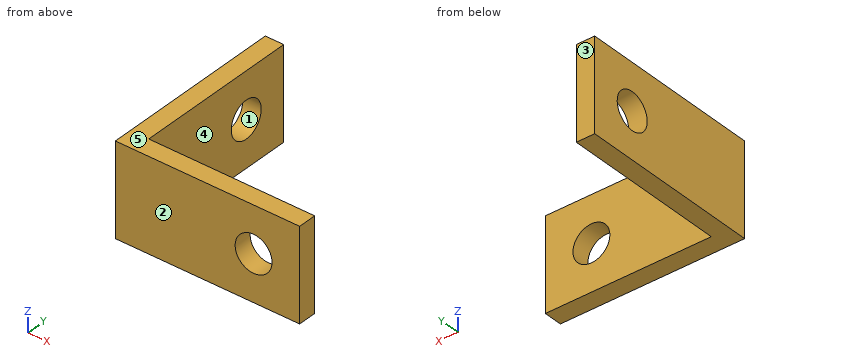
from build123d import *

# Parameters (mm, degrees)
SKETCH1_W           = 2
SKETCH1_H           = 18
SKETCH1_H_2         = 2
SKETCH1_W_2         = 18
BOSS_EXTRUDE2_DEPTH = 10
SKETCH3_R           = 2
CUT_EXTRUDE1_DEPTH  = 3
SKETCH4_R           = 2
CUT_EXTRUDE2_DEPTH  = 3


with BuildPart() as part:
    # Sketch1 → Boss-Extrude2 (new body)
    with BuildSketch(Plane.XY):
        with Locations((-8.840572317, 11)):
            Rectangle(SKETCH1_W, SKETCH1_H)
        with Locations((-8.840572317, 1)):
            Rectangle(SKETCH1_W, SKETCH1_H_2)
        with Locations((1.159427683, 1)):
            Rectangle(SKETCH1_W_2, SKETCH1_H_2)
    extrude(amount=BOSS_EXTRUDE2_DEPTH)

    # Sketch3 → Cut-Extrude1 (cut, through all)
    with BuildSketch(Plane(origin=(0, 2, 0), x_dir=(1, 0, 0), z_dir=(0, 1, 0))):
        with Locations((5.159427683, -5)):
            Circle(SKETCH3_R)
    extrude(amount=-CUT_EXTRUDE1_DEPTH, mode=Mode.SUBTRACT)

    # Sketch4 → Cut-Extrude2 (cut, through all)
    with BuildSketch(Plane(origin=(-7.840572317, 0, 0), x_dir=(0, 0, -1), z_dir=(1, 0, 0))):
        with Locations((-5, 15)):
            Circle(SKETCH4_R)
    extrude(amount=-CUT_EXTRUDE2_DEPTH, mode=Mode.SUBTRACT)


solid = part.part
Could you check a few things on this model? Use its own coordinates, in mm. Face numbers are marked on the shaded views. A direction names the side the tool comes from. Coordinates: 2 decimals unless noted, no trailing zeros. Loops run counter-clockwise (first coordinate to the right, second up) from the corner with the lowest first, then second, coordinate; pieces in that order, holes last.
1. Imagine slicing it at D-D (x = -6.5). Please give me the cut outline in (y, z), and give its area (3 significant figures).
2. For P1, Ø3, axis at y = 11, z = 6.5, coming from the +X side; P2, Ø12, axis at x = 4.5, y = 6, coming from the +Z side, each with a flat end and sliding along its axis, tell me the tip position at first contact or that it passes through.
3. Imagine slicing it at A-A (z = 5). Please give me the cut outline in (x, y), and give its area (3 significant figures).
4. Imagine slicing it at C-C (z = 8.25). Please give me the cut outline in (x, y), and give its area (3 significant figures).
5. We'd pull the mould along Y, two halves only. Please class the marked faces 1, 2 and 3: released by +Y, released by -Y, zero draft, split by the parting line, or undercut.
6. I need wall thicknesses on L1, parallel to X at y = 1.25, z = 5; L2, parallel to Y at x = -8.5, z = 5; L3, parallel to X at y = 19.25, z = 0.75. Which ranges of each line are inside material? Lowest first, please.
7. For the marked faces 4 and 5, which set-ups out of +Z, -Z, +X, -X, +Y, -Y let a thin tool reach every point of the face, with its end or its side?
8. Imagine slicing it at B-B (y = 15). Please give me the cut outline in (x, z).
Computed values:
1. outline: (0, 0) - (2, 0) - (2, 10) - (0, 10) - close
1. area: 20.0 mm2
2. P1: stops at x = -7.84
2. P2: stops at z = 10
3. outline: (-9.84, 0) - (3.16, 0) - (3.16, 2) - (-7.84, 2) - (-7.84, 13) - (-9.84, 13) - close; (-9.84, 17) - (-7.84, 17) - (-7.84, 20) - (-9.84, 20) - close; (7.16, 0) - (10.16, 0) - (10.16, 2) - (7.16, 2) - close
3. area: 60.0 mm2
4. outline: (-9.84, 0) - (10.16, 0) - (10.16, 2) - (-7.84, 2) - (-7.84, 20) - (-9.84, 20) - close
4. area: 76.0 mm2
5. face 1: undercut
5. face 2: released by -Y
5. face 3: released by +Y
6. L1: x = -9.84 to 3.16, 7.16 to 10.16
6. L2: y = 0 to 13, 17 to 20
6. L3: x = -9.84 to -7.84
7. face 4: +Z, -Z, +X, +Y
7. face 5: +Z, +X, -X, +Y, -Y
8. outline: (-9.84, 0) - (-7.84, 0) - (-7.84, 3) - (-9.84, 3) - close; (-9.84, 7) - (-7.84, 7) - (-7.84, 10) - (-9.84, 10) - close
